Source: CAD feature listing. Evaluate the final solid. Frame: model axes, mm. Coordinates: 2 decimals unless noted, no trailing zeros. Write each loop counter-clockwise with the first axis right and the second up, starting at its lowest first coordinate (ties: lowest second). Pieces come first, ordered by that corner, then holes. Notation, with made-up numbers: M 83.5,87 L 124.5,87 A11 ccw 124.5,107 Z; hole C 51.5,23.5 d9. An arc over 180 degrees is marked long. One line per item, written item: value. Start each with the question number.
Item 1: Cut plane A-A, the plane x = 78. Output: boundary loops of the cut face in (y, z), then the cut area to 3 significant figures.
Item 2: Cut plane C-C, the plane z = 0.35. State how many separate pieces and enclosed holes the cut face has, then the cut area to 3 significant figures.
Item 3: Ray query, L1, parallel to X at y = 7, z = 0.7; L2, parallel to Y at x = 3, z = 0.65; L3, parallel to X at y = 96, z = 0.7. Return the intervals inside material, ascending. Write a range as from..to.
Item 4: Cut plane B-B, the plane y = 81. Output: boundary loops of the cut face in (x, z), then the cut area to 3 significant figures.
Item 5: Pin query (flat end, axial travel): P1, Ø1, axis at x = 152.5, y = 43, coming from the -Z side. Return the tip coordinate at first contact, or that it passes through.
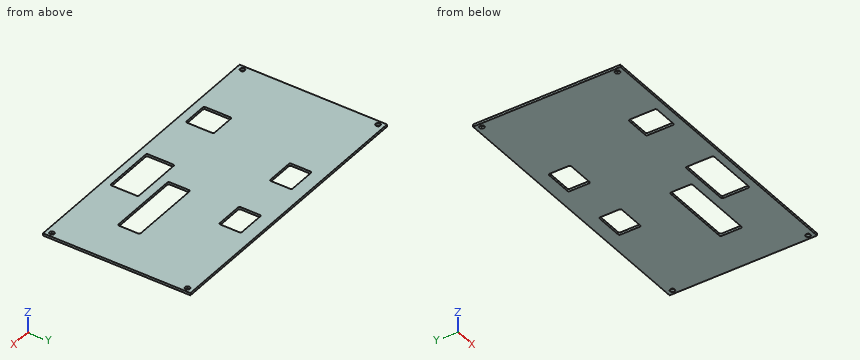
```python
from build123d import *

# Parameters (mm, degrees)
ESQUISSE1_W             = 194
ESQUISSE1_H             = 100
BOSS_EXTRU_1_DEPTH      = 1.6
ESQUISSE2_R             = 1.6
ENL_V_MAT_EXTRU_1_DEPTH = 1.6


with BuildPart() as part:
    # Esquisse1 → Boss.-Extru.1 (new body)
    with BuildSketch(Plane.XY):
        with Locations((97, 50)):
            Rectangle(ESQUISSE1_W, ESQUISSE1_H)
    extrude(amount=BOSS_EXTRU_1_DEPTH)

    # Esquisse2 → Enlèv. mat.-Extru.1 (cut)
    with BuildSketch(Plane.XY.offset(1.6)):
        with Locations((3, 96)):
            Circle(ESQUISSE2_R)
        with Locations((191, 96)):
            Circle(ESQUISSE2_R)
        with Locations((191, 4)):
            Circle(ESQUISSE2_R)
        with Locations((3, 4)):
            Circle(ESQUISSE2_R)
        with BuildLine():
            Line((45, 25), (61, 25))
            ThreePointArc((61, 25), (61.707106781, 24.707106781), (62, 24))
            Line((62, 24), (62, 7))
            ThreePointArc((62, 7), (61.707106781, 6.292893219), (61, 6))
            Line((61, 6), (45, 6))
            ThreePointArc((45, 6), (44.292893219, 6.292893219), (44, 7))
            Line((44, 7), (44, 24))
            ThreePointArc((44, 24), (44.292893219, 24.707106781), (45, 25))
        make_face()
        with BuildLine():
            Line((62, 91), (80, 91))
            ThreePointArc((80, 91), (80.707106781, 90.707106781), (81, 90))
            Line((81, 90), (81, 77))
            ThreePointArc((81, 77), (80.707106781, 76.292893219), (80, 76))
            Line((80, 76), (62, 76))
            ThreePointArc((62, 76), (61.292893219, 76.292893219), (61, 77))
            Line((61, 77), (61, 90))
            ThreePointArc((61, 90), (61.292893219, 90.707106781), (62, 91))
        make_face()
        with BuildLine():
            Line((112, 91), (130, 91))
            ThreePointArc((130, 91), (130.707106781, 90.707106781), (131, 90))
            Line((131, 90), (131, 77))
            ThreePointArc((131, 77), (130.707106781, 76.292893219), (130, 76))
            Line((130, 76), (112, 76))
            ThreePointArc((112, 76), (111.292893219, 76.292893219), (111, 77))
            Line((111, 77), (111, 90))
            ThreePointArc((111, 90), (111.292893219, 90.707106781), (112, 91))
        make_face()
        with BuildLine():
            Line((115, 45), (163, 45))
            ThreePointArc((163, 45), (163.707106781, 44.707106781), (164, 44))
            Line((164, 44), (164, 31))
            ThreePointArc((164, 31), (163.707106781, 30.292893219), (163, 30))
            Line((163, 30), (115, 30))
            ThreePointArc((115, 30), (114.292893219, 30.292893219), (114, 31))
            Line((114, 31), (114, 44))
            ThreePointArc((114, 44), (114.292893219, 44.707106781), (115, 45))
        make_face()
        with BuildLine():
            Line((100, 24), (134, 24))
            ThreePointArc((134, 24), (134.707106781, 23.707106781), (135, 23))
            Line((135, 23), (135, 6))
            ThreePointArc((135, 6), (134.707106781, 5.292893219), (134, 5))
            Line((134, 5), (100, 5))
            ThreePointArc((100, 5), (99.292893219, 5.292893219), (99, 6))
            Line((99, 6), (99, 23))
            ThreePointArc((99, 23), (99.292893219, 23.707106781), (100, 24))
        make_face()
    extrude(amount=-ENL_V_MAT_EXTRU_1_DEPTH, mode=Mode.SUBTRACT)


solid = part.part
```
From the geometry:
1. outline: M 0,0 L 76,0 L 76,1.6 L 0,1.6 Z; M 91,0 L 100,0 L 100,1.6 L 91,1.6 Z
1. area: 136 mm²
2. separate pieces: 1
2. enclosed holes: 9
2. area: 17,000 mm²
3. L1: x = 0..44, 62..99, 135..194
3. L2: y = 0..2.4, 5.6..94.4, 97.6..100
3. L3: x = 0..1.4, 4.6..189.4, 192.6..194
4. outline: M 0,0 L 61,0 L 61,1.6 L 0,1.6 Z; M 81,0 L 111,0 L 111,1.6 L 81,1.6 Z; M 131,0 L 194,0 L 194,1.6 L 131,1.6 Z
4. area: 246 mm²
5. P1: passes through
